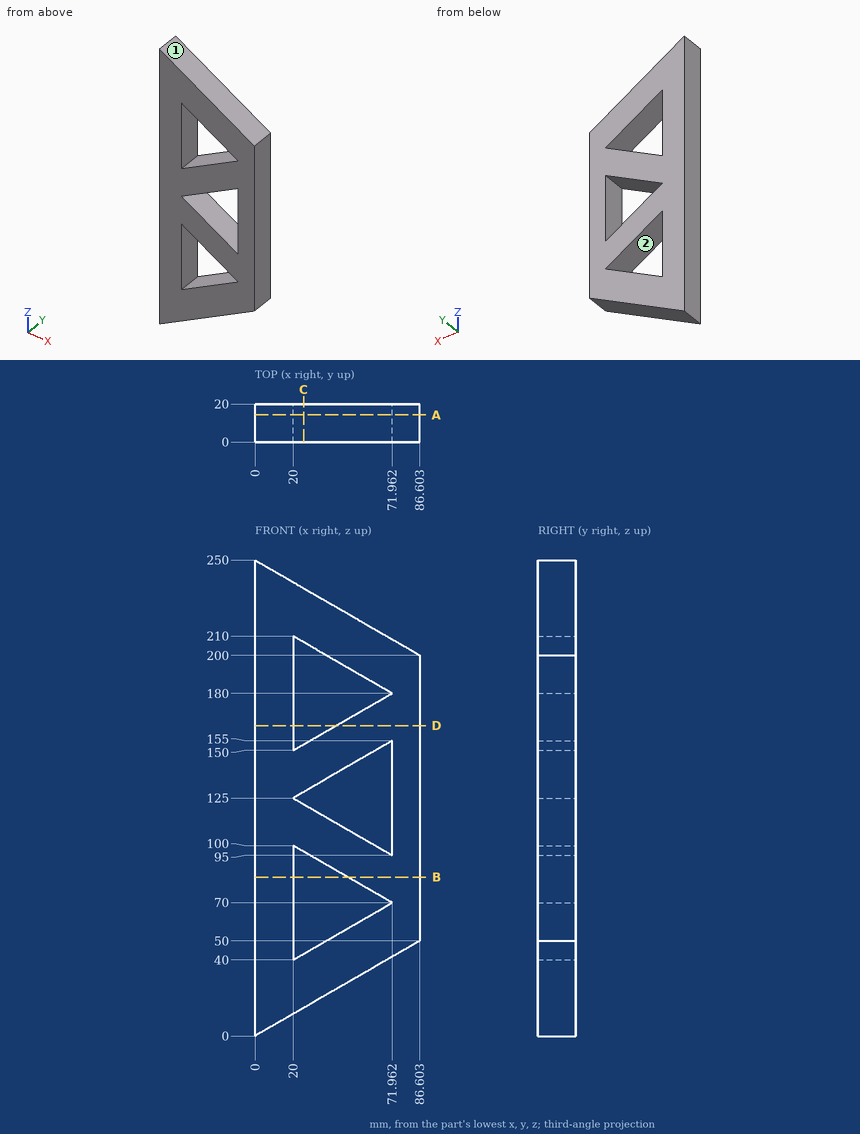
For this review, use the dimensioned drawing (mm, ordinates from the lowest corner) and the shaded views. A direction names the side the tool comes from. Give positions to 0.01 mm unless a question says otherwise; leave off trailing zeros. Order: outer loops, then holes, each group sorted by start corner. A loop starts at its lowest first (then second) coordinate and runs counter-clockwise, first axis right, second up.
1. Tool access review of the marked faces 1 and 2: name each direction out of +Z, -Z, +X, -X, +Y, -Y from which nothing blocks a thin tool from reaching the whole face with its end or side.
Solution:
face 1: +Z, +X, +Y, -Y
face 2: +Y, -Y
2. To check wall thickness, follow L1, parallel to Z at x = 64.5, y = 9.75; L2, parallel to X at y = 6.75, z = 70 (1 decimal); L3, parallel to Z at x = 22, y = 8 (1 decimal). State the ranges of each line that lie inside material, in increasing order.
Solution:
L1: z = 37.24 to 65.69, 74.31 to 99.31, 150.69 to 175.69, 184.31 to 212.76
L2: x = 0 to 20, 72 to 86.6
L3: z = 12.7 to 41.2, 98.8 to 123.8, 126.2 to 151.2, 208.8 to 237.3
3. Add section A-A, the plane y = 14.25. State the section outline as (x, z) points, then the cut area to 3 significant figures.
Solution:
outline: (0, 0) - (86.6, 50) - (86.6, 200) - (0, 250) - close; hole (20, 40) - (71.96, 70) - (20, 100) - close; hole (20, 125) - (71.96, 95) - (71.96, 155) - close; hole (20, 150) - (71.96, 180) - (20, 210) - close
area: 12,600 mm2
4. For pin 1 Ø1 at (y, z) = (13, 222.5) entering from +X (1 decimal); pin 2 Ø10 at (x, y) = (36, 3.5) entering from -Z, all flat-tipped, find the tip position at first contact; note any pin that passes through.
Solution:
pin 1: stops at x = 48.5
pin 2: stops at z = 17.9
5. Add section B-B, the plane z = 83.5. State the section outline as (x, y) points.
Solution:
outline: (0, 0) - (20, 0) - (20, 20) - (0, 20) - close; (48.58, 0) - (86.6, 0) - (86.6, 20) - (48.58, 20) - close
6. Add section D-D, the plane z = 163. State the section outline as (x, y) points.
Solution:
outline: (0, 0) - (20, 0) - (20, 20) - (0, 20) - close; (42.52, 0) - (86.6, 0) - (86.6, 20) - (42.52, 20) - close
7. Add section C-C, the plane x = 25.5. State the section outline as (y, z) points (1 decimal), then the cut area to 3 significant figures.
Solution:
outline: (0, 14.7) - (20, 14.7) - (20, 43.2) - (0, 43.2) - close; (0, 96.8) - (20, 96.8) - (20, 121.8) - (0, 121.8) - close; (0, 128.2) - (20, 128.2) - (20, 153.2) - (0, 153.2) - close; (0, 206.8) - (20, 206.8) - (20, 235.3) - (0, 235.3) - close
area: 2,140 mm2
